```python
from build123d import *

# Parameters (mm, degrees)
ESBO_O1_W                 = 100
ESBO_O1_H                 = 43
RESSALTO_EXTRUS_O1_DEPTH  = 1.5
ESBO_O2_R                 = 1.5
CORTE_EXTRUS_O1_DEPTH     = 4
SKETCH7_W                 = 13.5
SKETCH7_H                 = 9.5
CUT_EXTRUDE6_DEPTH        = 2.5
CUT_EXTRUDE6_DEPTH_BACK   = 2.5
SKETCH8_W                 = 3
SKETCH8_H                 = 34.5
BOSS_EXTRUDE1_DEPTH       = 1.5
FILLET3_R                 = 2
FILLET4_R                 = 5
SKETCH9_R                 = 1.5
SKETCH9_W                 = 11.5
SKETCH9_H                 = 3
CORTE_GY_53LDK_DEPTH      = 2.5
CORTE_GY_53LDK_DEPTH_BACK = 2.5


with BuildPart() as part:
    # Esboço1 → Ressalto-extrusão1 (new body, symmetric)
    with BuildSketch(Plane.XY):
        Rectangle(ESBO_O1_W, ESBO_O1_H)
    extrude(amount=RESSALTO_EXTRUS_O1_DEPTH, both=True)

    # Esboço2 → Corte-extrusão1 (cut, through all)
    with BuildSketch(Plane.XY.offset(1.5)):
        with Locations((-33, -17)):
            Circle(ESBO_O2_R)
        with Locations((33, -17)):
            Circle(ESBO_O2_R)
        Polygon((-20, -15.5), (-7.5, -15.5), (-7.5, -12.5), (7.5, -12.5), (7.5, -15.5), (20, -15.5), (20, -18.5), (7.5, -18.5), (7.5, -21.5), (-7.5, -21.5), (-7.5, -18.5), (-20, -18.5), align=None)
    extrude(amount=-CORTE_EXTRUS_O1_DEPTH, mode=Mode.SUBTRACT)

    # Sketch7 → Cut-Extrude6 (cut, two sides)
    with BuildSketch(Plane.XY) as cut_extrude6_sk:
        with Locations((-11.75, 0)):
            Rectangle(SKETCH7_W, SKETCH7_H)
        with Locations((11.75, 0)):
            Rectangle(SKETCH7_W, SKETCH7_H)
    extrude(amount=CUT_EXTRUDE6_DEPTH, mode=Mode.SUBTRACT)
    extrude(cut_extrude6_sk.sketch, amount=-CUT_EXTRUDE6_DEPTH_BACK, mode=Mode.SUBTRACT)

    # Sketch8 → Boss-Extrude1 (add, symmetric)
    with BuildSketch(Plane.XY):
        with Locations((-51.5, 4.25)):
            Rectangle(SKETCH8_W, SKETCH8_H)
        with Locations((51.5, 4.25)):
            Rectangle(SKETCH8_W, SKETCH8_H)
    extrude(amount=BOSS_EXTRUDE1_DEPTH, both=True)

    # Fillet3
    fillet3_edges = [part.edges().sort_by_distance(p)[0] for p in [
        (-7.5, -21.5, 0),
        (-7.5, -12.5, 0),
        (7.5, -12.5, 0),
        (7.5, -21.5, 0),
    ]]
    fillet(fillet3_edges, radius=FILLET3_R)

    # Fillet4
    fillet4_edges = [part.edges().sort_by_distance(p)[0] for p in [
        (53, 21.5, 0),
        (-53, 21.5, 0),
    ]]
    fillet(fillet4_edges, radius=FILLET4_R)

    # Sketch9 → Corte Gy-53LDK (cut, two sides)
    with BuildSketch(Plane.XY) as corte_gy_53ldk_sk:
        with Locations((-41.25, 6.7)):
            Circle(SKETCH9_R)
        with Locations((46.25, 6.7)):
            Circle(SKETCH9_R)
        with Locations((-43.75, 16)):
            Rectangle(SKETCH9_W, SKETCH9_H)
        with Locations((43.75, 16)):
            Rectangle(SKETCH9_W, SKETCH9_H)
    extrude(amount=CORTE_GY_53LDK_DEPTH, mode=Mode.SUBTRACT)
    extrude(corte_gy_53ldk_sk.sketch, amount=-CORTE_GY_53LDK_DEPTH_BACK, mode=Mode.SUBTRACT)


solid = part.part
```
Here's how the part is built. I have some questions about the finished solid (model axes, mm). A direction names the side the tool comes from. Give positions to 0.01 mm unless a question says otherwise; leave off trailing zeros. Write each loop counter-clockwise with the first axis right and the second up, starting at its lowest first coordinate (ties: lowest second). Pieces come first, ordered by that corner, then holes.
(1) Imagine slicing it at A-A, the plane x = -33. Write out the boundary of the cut face in (y, z), and give its area (3 significant figures).
Output values:
outline: (-21.5, -1.5) - (-18.5, -1.5) - (-18.5, 1.5) - (-21.5, 1.5) - close; (-15.5, -1.5) - (21.5, -1.5) - (21.5, 1.5) - (-15.5, 1.5) - close
area: 120 mm2
(2) On a 3-axis mill with a long thin cutter (end or side, diameter ignored), from which of +Z, -Z, +X, -X, +Y, -Y can I reach the whole of each face in a straight line? I mean faces 1 (the face through (0, -12.5, 0)), 2 (the face through (-12, 4.75, 0)), 3 (the face through (50, -17, 0)). Say none if no direction works.
Output values:
face 1: +Z, -Z, -Y
face 2: +Z, -Z
face 3: +Z, -Z, +X, -Y
(3) If I drill on L1, parallel to X at y = 3.5, z = -0.2; L2, parallel to Y at x = -41.25, z = -1.1; L3, parallel to X at y = 6.7, z = 1.1, over which ranges is the centre line in solid material (lowest first)?
Output values:
L1: x = -53 to -18.5, -5 to 5, 18.5 to 53
L2: y = -21.5 to 5.2, 8.2 to 14.5, 17.5 to 21.5
L3: x = -53 to -42.75, -39.75 to 44.75, 47.75 to 53
(4) Imagine slicing it at B-B, the plane y = -17. Write out the boundary of the cut face in (x, z).
Output values:
outline: (-50, -1.5) - (-34.5, -1.5) - (-34.5, 1.5) - (-50, 1.5) - close; (-31.5, -1.5) - (-20, -1.5) - (-20, 1.5) - (-31.5, 1.5) - close; (20, -1.5) - (31.5, -1.5) - (31.5, 1.5) - (20, 1.5) - close; (34.5, -1.5) - (50, -1.5) - (50, 1.5) - (34.5, 1.5) - close
(5) Imagine slicing it at D-D, the plane x = 46.25. Write out the boundary of the cut face in (y, z).
Output values:
outline: (-21.5, -1.5) - (5.2, -1.5) - (5.2, 1.5) - (-21.5, 1.5) - close; (8.2, -1.5) - (14.5, -1.5) - (14.5, 1.5) - (8.2, 1.5) - close; (17.5, -1.5) - (21.5, -1.5) - (21.5, 1.5) - (17.5, 1.5) - close
(6) Imagine slicing it at C-C, the plane y = 6.7. Write out the boundary of the cut face in (x, z).
Output values:
outline: (-53, -1.5) - (-42.75, -1.5) - (-42.75, 1.5) - (-53, 1.5) - close; (-39.75, -1.5) - (44.75, -1.5) - (44.75, 1.5) - (-39.75, 1.5) - close; (47.75, -1.5) - (53, -1.5) - (53, 1.5) - (47.75, 1.5) - close
(7) Thinking about a two-plate mould opening in X: for faces 4 (the face through (-6.9, -13.07, -0.02)), 5 (the face through (-1, 0, -1.5)), 6 (the face through (53, 2, 0)), which applies, pulls with the +X half, pulls with the -X half, needs draft (parallel to the pull), parting line crosses it, or undercut?
Output values:
face 4: undercut
face 5: needs draft
face 6: pulls with the +X half
